Autodesk Inventor part; units mm, degrees
ref_plane "XZ Plane" through (0, 0, 0) normal (0, 1, 0) x (-1, 0, 0)
ref_plane "XY Plane" through (0, 0, 0) normal (0, 0, 1) x (1, 0, 0)
sketch "Sketch1" plane through (0, 0, 0) normal (0, 0, 1) x (1, 0, 0)
  circle A0 centre (0, 0) radius 1
  dimension "d0" = 2
extrude "Extrusion1" add sketch "Sketch1" against normal blind 40
ref_plane "Work Plane1" through (0, 0, -40) normal (0, 0, -1) x (-1, 0, 0)
ref_plane "Work Plane3" through (0, 0, -40) normal (0.7071, 0, 0.7071) x (0, -1, 0)
ref_plane "Work Plane2" through (0, 0, -40) normal (1, 0, 0) x (0, 1, 0)
sketch "Sketch2" plane through (0, 0, -40) normal (0.7071, 0, 0.7071) x (0, -1, 0)
  ellipse E0 centre (0, 0) end of major axis (-1, 0) minor radius 0.7071
  circle A0 centre (0, 0) radius 1
  point P0 (0, -28.2843)
extrude "Extrusion2" add sketch "Sketch2" along normal blind 40
ref_plane "Work Plane4" through (28.2843, 0, -11.7157) normal (0, 0, -1) x (-1, 0, 0)
sketch "Sketch3" plane through (28.2843, 0, -11.7157) normal (0, 0, -1) x (-1, 0, 0)
  ellipse E0 centre (0, 0) end of major axis (0, 1) minor radius 0.7071
  circle A0 centre (0, 0) radius 1
  point P0 (28.2843, 0)
extrude "Extrusion3" add sketch "Sketch3" along normal blind 40
ref_plane "Work Plane5" through (0, 0, -40) normal (0.3827, 0, 0.9239) x (0, -1, 0)
sketch "Sketch4" plane through (0, 0, -40) normal (0.3827, 0, 0.9239) x (0, -1, 0)
  circle A0 centre (0, 0) radius 2.8545
  point P0 (0, -15.3073)
extrude "Extrusion4" add sketch "Sketch4" along normal blind 1
ref_plane "Work Plane6" through (28.2843, 0, -11.7157) normal (0.3827, 0, 0.9239) x (0.9239, 0, -0.3827)
sketch "Sketch5" plane through (28.2843, 0, -11.7157) normal (0.3827, 0, 0.9239) x (0.9239, 0, -0.3827)
  circle A0 centre (0, 0) radius 2.6859
  point P0 (-30.6147, 0)
extrude "Extrusion5" add sketch "Sketch5" against normal blind 1
ref_plane "Work Plane7" through (28.2843, 0, -26.2157) normal (0, 0, -1) x (-1, 0, 0)
sketch "Sketch6" plane through (28.2843, 0, -26.2157) normal (0, 0, -1) x (-1, 0, 0)
  ellipse E0 centre (0, 0) end of major axis (0, 2.6859) minor radius 2.4814
  line L0 (-2.1727, -1.2973) -> (2.1727, -1.2973)
  line L1 (2.1727, -1.2973) -> (2.1727, 1.2973)
  line L2 (2.1727, 1.2973) -> (-2.1727, 1.2973)
  line L3 (-2.1727, 1.2973) -> (-2.1727, -1.2973)
  line L4 (0, -1) -> (0, 1)
  line L5 (-2.1727, -1.2973) -> (2.1727, 1.2973) construction
  line L6 (2.1727, -1.2973) -> (-2.1727, 1.2973) construction
  point P0 (28.2843, 0)
  point P1 (0, 0)
extrude "Extrusion6" add sketch "Sketch6" along normal blind 1 contours L2 L1 L0 L3
properties part number "00_Beam_Ocular_Detectoin"
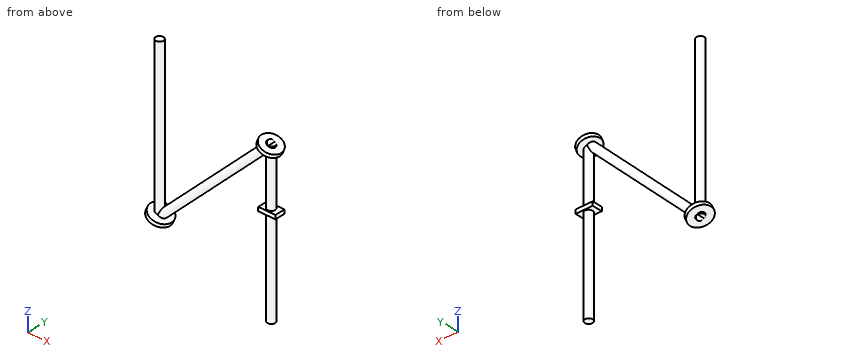
Input: part model. Units: mm. Frame: model coordinates. Coordinates: 2 decimals unless noted, no trailing zeros. Write each loop counter-clockwise with the first axis right and the second up, starting at its lowest first coordinate (ties: lowest second). Pieces come first, ordered by that corner, then holes. Notation, with made-up numbers: M 88,-3.5 L 98,-3.5 A24 cw 98,7.5 Z; hole C 78,87.5 d11. An arc over 180 degrees is marked long. Answer as a JSON object with one key per item and string values. Group by question number.
(1) Contact query for flat-ended pins moving along their axis: P1, Ø5, axis at x = 9, z = -25, coming from the +Y side (3 decimals); P2, Ø1.1, axis at x = 29, y = 0, coming from the +Z side; P3, Ø1.1, axis at y = -0.5, z = -26.5, coming from the -X side; P4, Ø0.5, axis at x = 29, z = -27, coming from the +Y side. Output: stop coordinate, or through.
(2) Ray query, line 1 along X through (y, z) = (0.2, -28); line 2 along X through (y, z) = (0.4, -21.5); line 3 along X through (y, z) = (1.1, -27). Return the intervals inside material, ascending. Write a range as [from, to].
(3) Section B-B on z = -29.5. Give the number of separate pieces and of enclosed holes in the cut face, plus the area to 3 significant figures.
(4) Section A-A on z = -44. Output: boundary loops of the cut face in (x, y).
Result set:
{
 "1": {"P1": "passes through", "P2": "stops at z = -11.72", "P3": "stops at x = -1", "P4": "stops at y = 1.3"},
 "2": {"line 1": "x = [-0.98, 0.98], [10.61, 13.39], [27.3, 29.26]", "line 2": "x = [-0.92, 0.92], [17.2, 19.8], [27.37, 29.2]", "line 3": "x = [26.11, 30.46]"},
 "3": {"separate pieces": "3", "enclosed holes": "0", "area": "10.7 mm2"},
 "4": {"outline": "C 28.28,0 d2"}
}
